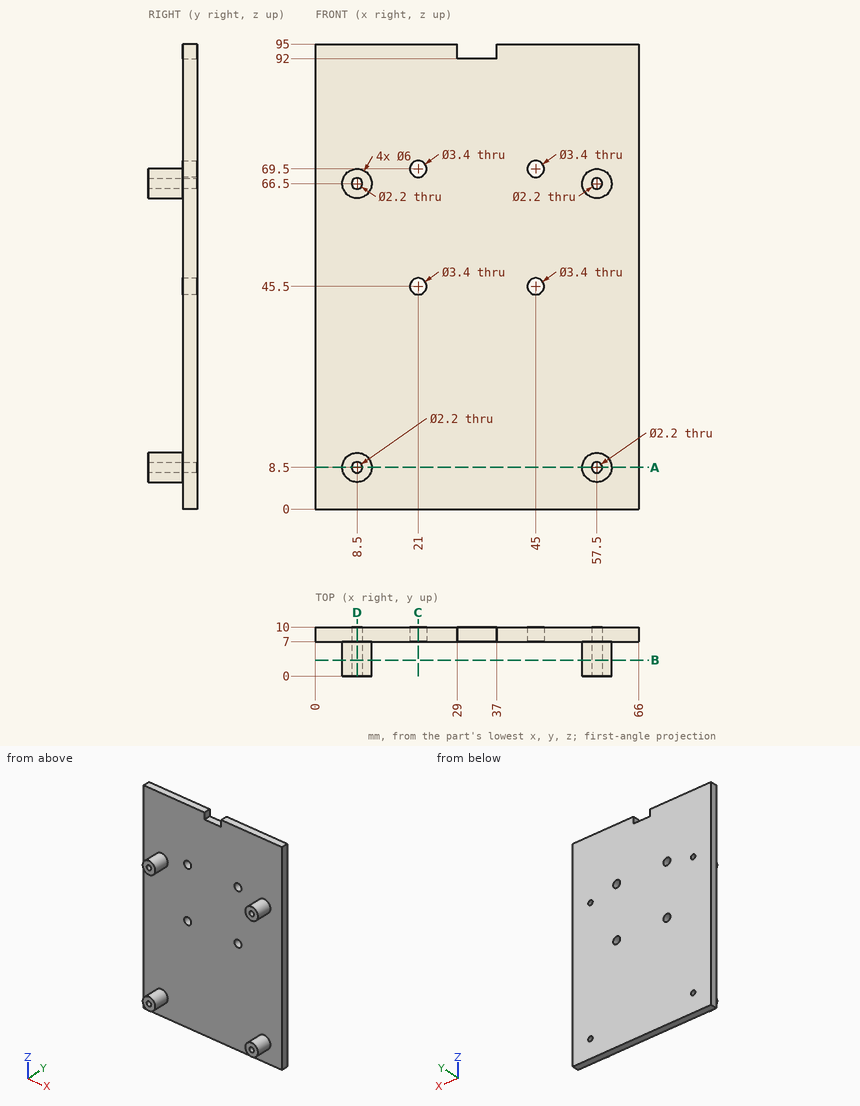
The drawing under review shows one solid part. Ordinate dimensions are in mm from its lowest x, y, z. Coordinates: 2 decimals unless noted, no trailing zeros. Write each loop counter-clockwise with the first axis right and the second up, starting at its lowest first coordinate (ties: lowest second). Pieces come first, ordered by that corner, then holes.
1) Insertion check: pin 1 (5 mm diameter, centred on y = 1.5, z = 66, fed in from -X); pin 2 (1.5 mm diameter, centred on x = 36, y = 7.5, fed in from +Z); pin 3 (4.5 mm diameter, centred on x = 21, z = 69.5, fed in from -Y). Each pin has a flat end and moves straight along its axis. Give the tip position at first contact, or say it passes through.
2) Add section C-C (x = 21). Write out the cut boundary in (y, z).
3) To check wall thickness, follow L1, parallel to Z at x = 57.5, y = 6.75; L2, parallel to Z at x = 21, y = 9.45; L3, parallel to X at y = 6.5, z = 8.5. State the ranges of each line that lie inside material, in increasing order.
4) Add section D-D (x = 8.5). Write out the cut boundary in (y, z), plus the area to 3 significant figures.
5) Add section A-A (z = 8.5). Write out the cut boundary in (x, y).
6) Add section B-B (y = 3.25). Write out the cut boundary in (x, z).
Check result:
1. pin 1: stops at x = 5.5
1. pin 2: stops at z = 92
1. pin 3: stops at y = 7
2. outline: (7, 0) - (10, 0) - (10, 43.8) - (7, 43.8) - close; (7, 47.2) - (10, 47.2) - (10, 67.8) - (7, 67.8) - close; (7, 71.2) - (10, 71.2) - (10, 95) - (7, 95) - close
3. L1: z = 5.5 to 7.4, 9.6 to 11.5, 63.5 to 65.4, 67.6 to 69.5
3. L2: z = 0 to 43.8, 47.2 to 67.8, 71.2 to 95
3. L3: x = 5.5 to 7.4, 9.6 to 11.5, 54.5 to 56.4, 58.6 to 60.5
4. outline: (0, 5.5) - (7, 5.5) - (7, 0) - (10, 0) - (10, 7.4) - (0, 7.4) - close; (0, 9.6) - (10, 9.6) - (10, 65.4) - (0, 65.4) - (0, 63.5) - (7, 63.5) - (7, 11.5) - (0, 11.5) - close; (0, 67.6) - (10, 67.6) - (10, 95) - (7, 95) - (7, 69.5) - (0, 69.5) - close
4. area: 325 mm2
5. outline: (0, 7) - (5.5, 7) - (5.5, 0) - (7.4, 0) - (7.4, 10) - (0, 10) - close; (9.6, 0) - (11.5, 0) - (11.5, 7) - (54.5, 7) - (54.5, 0) - (56.4, 0) - (56.4, 10) - (9.6, 10) - close; (58.6, 0) - (60.5, 0) - (60.5, 7) - (66, 7) - (66, 10) - (58.6, 10) - close
6. outline: circle Ø6 at (8.5, 8.5); circle Ø6 at (8.5, 66.5); circle Ø6 at (57.5, 8.5); circle Ø6 at (57.5, 66.5); hole circle Ø2.2 at (8.5, 8.5); hole circle Ø2.2 at (8.5, 66.5); hole circle Ø2.2 at (57.5, 8.5); hole circle Ø2.2 at (57.5, 66.5)
